CAD build for the part. Positions are in the model's coordinates, mm. Coordinates: 2 decimals unless noted, no trailing zeros. Order: outer loops, then holes, each group sorted by start corner. A loop starts at its lowest first (then second) coordinate and runs counter-clockwise, first axis right, second up. Notation, with made-up numbers: M -28.75,61.25 L -18.75,61.25 A24 cw -18.75,87.25 Z; hole C 86,76 d7. An arc over 180 degrees is marked long. Write item = value, one per line.
from build123d import *

# Parameters (mm, degrees)
CYLINDER115_R          = 1.6
CYLINDER115_DEPTH      = 10
CYLINDER116_R          = 1.6
CYLINDER116_DEPTH      = 10
CYLINDER117_R          = 1.6
CYLINDER117_DEPTH      = 10
CYLINDER114_R          = 1.6
CYLINDER114_DEPTH      = 10
CYLINDER111_R          = 2
CYLINDER111_DEPTH      = 10
CYLINDER110_R          = 2
CYLINDER110_DEPTH      = 10
CYLINDER113_R          = 1.75
CYLINDER113_DEPTH      = 10
CYLINDER112_R          = 1.75
CYLINDER112_DEPTH      = 10
CYLINDER104_R          = 2
CYLINDER104_DEPTH      = 10
CYLINDER105_R          = 2
CYLINDER105_DEPTH      = 10
CYLINDER106_R          = 2
CYLINDER106_DEPTH      = 10
CYLINDER107_R          = 2
CYLINDER107_DEPTH      = 10
CYLINDER109_R          = 24
CYLINDER109_DEPTH      = 7
CYLINDER108_R          = 40
CYLINDER108_DEPTH      = 5
CUT014_PLACEMENT_ANGLE = 1


with BuildPart() as obj1:
    # Cylinder115 → Cylinder115 (new body)
    with BuildSketch(Plane(origin=(40, 0, 65), x_dir=(1, 0, 0), z_dir=(0, 0, 1))):
        Circle(CYLINDER115_R)
    extrude(amount=CYLINDER115_DEPTH)


with BuildPart() as obj2:
    # Cylinder116 → Cylinder116 (new body)
    with BuildSketch(Plane(origin=(5, 35, 65), x_dir=(1, 0, 0), z_dir=(0, 0, 1))):
        Circle(CYLINDER116_R)
    extrude(amount=CYLINDER116_DEPTH)


with BuildPart() as obj3:
    # Cylinder117 → Cylinder117 (new body)
    with BuildSketch(Plane(origin=(5, -35, 65), x_dir=(1, 0, 0), z_dir=(0, 0, 1))):
        Circle(CYLINDER117_R)
    extrude(amount=CYLINDER117_DEPTH)


with BuildPart() as fusion037:
    # Cylinder114 → Cylinder114 (new body)
    with BuildSketch(Plane(origin=(-30, 0, 65), x_dir=(1, 0, 0), z_dir=(0, 0, 1))):
        Circle(CYLINDER114_R)
    extrude(amount=CYLINDER114_DEPTH)

    # Fusion037: union obj1, obj2, obj3
    add(obj1.part)
    add(obj2.part)
    add(obj3.part)


with BuildPart() as wirecut007:
    # Cylinder111 → Cylinder111 (new body)
    with BuildSketch(Plane(origin=(15, 0, 70), x_dir=(1, 0, 0), z_dir=(0, 0, 1))):
        Circle(CYLINDER111_R)
    extrude(amount=CYLINDER111_DEPTH)


with BuildPart() as wirecuts003:
    # Cylinder110 → Cylinder110 (new body)
    with BuildSketch(Plane(origin=(-5, 0, 70), x_dir=(1, 0, 0), z_dir=(0, 0, 1))):
        Circle(CYLINDER110_R)
    extrude(amount=CYLINDER110_DEPTH)

    # Fusion033: union wireCUt007
    add(wirecut007.part)


with BuildPart() as m3cuts007:
    # Cylinder113 → Cylinder113 (new body)
    with BuildSketch(Plane(origin=(5, 9, 70), x_dir=(1, 0, 0), z_dir=(0, 0, 1))):
        Circle(CYLINDER113_R)
    extrude(amount=CYLINDER113_DEPTH)


with BuildPart() as m3cute003:
    # Cylinder112 → Cylinder112 (new body)
    with BuildSketch(Plane(origin=(5, -9, 70), x_dir=(1, 0, 0), z_dir=(0, 0, 1))):
        Circle(CYLINDER112_R)
    extrude(amount=CYLINDER112_DEPTH)

    # Fusion034: union m3Cuts007
    add(m3cuts007.part)


with BuildPart() as cylinder104:
    # Cylinder104 → Cylinder104 (new body)
    with BuildSketch(Plane(origin=(0, -21, 0), x_dir=(1, 0, 0), z_dir=(0, 0, 1))):
        Circle(CYLINDER104_R)
    extrude(amount=CYLINDER104_DEPTH)


with BuildPart() as m3heatsetcuts009:
    # Cylinder105 → Cylinder105 (new body)
    with BuildSketch(Plane(origin=(20, -21, 0), x_dir=(1, 0, 0), z_dir=(0, 0, 1))):
        Circle(CYLINDER105_R)
    extrude(amount=CYLINDER105_DEPTH)

    # Fusion030: union Cylinder104
    add(cylinder104.part)


with BuildPart() as m3heatsetcuts009_1:
    # Fusion030 placement: moved
    add(m3heatsetcuts009.part.moved(Location((-5, 38.5, 70))))


with BuildPart() as cylinder106:
    # Cylinder106 → Cylinder106 (new body)
    with BuildSketch(Plane(origin=(0, -21, 0), x_dir=(1, 0, 0), z_dir=(0, 0, 1))):
        Circle(CYLINDER106_R)
    extrude(amount=CYLINDER106_DEPTH)


with BuildPart() as basecuts003:
    # Cylinder107 → Cylinder107 (new body)
    with BuildSketch(Plane(origin=(20, -21, 0), x_dir=(1, 0, 0), z_dir=(0, 0, 1))):
        Circle(CYLINDER107_R)
    extrude(amount=CYLINDER107_DEPTH)

    # Fusion031: union Cylinder106
    add(cylinder106.part)


with BuildPart() as basecuts003_1:
    # Fusion031 placement: moved
    add(basecuts003.part.moved(Location((-5, 3.5, 70))))

    # Fusion032: union m3HeatSetCuts009
    add(m3heatsetcuts009_1.part)

    # Fusion035: union wireCuts003, m3Cute003
    add(wirecuts003.part)
    add(m3cute003.part)


with BuildPart() as basecut003:
    # Cylinder109 → Cylinder109 (new body)
    with BuildSketch(Plane(origin=(5, 0, 74), x_dir=(1, 0, 0), z_dir=(0, 0, 1))):
        Circle(CYLINDER109_R)
    extrude(amount=CYLINDER109_DEPTH)


with BuildPart() as cut012:
    # Sphere004 → Sphere004 (revolve)
    with BuildSketch(Plane(origin=(5, 0, 74), x_dir=(1, 0, 0), z_dir=(0, -1, 0))):
        with BuildLine():
            ThreePointArc((29, 0), (28.841135, 3.031325), (28.36628, 6.029439))
            Line((28.36628, 6.029439), (0, 6.029439))
            Line((0, 6.029439), (0, 0))
            Line((0, 0), (29, 0))
        make_face()
    revolve(axis=Axis((5, 0, 74), (0, 0, 1)))

    # Cut012: cut baseCut003
    add(basecut003.part, mode=Mode.SUBTRACT)


with BuildPart() as lightmodule003:
    # Cylinder108 → Cylinder108 (new body)
    with BuildSketch(Plane(origin=(5, 0, 70), x_dir=(1, 0, 0), z_dir=(0, 0, 1))):
        Circle(CYLINDER108_R)
    extrude(amount=CYLINDER108_DEPTH)

    # Fusion036: union Cut012
    add(cut012.part)

    # Cut013: cut baseCUts003
    add(basecuts003_1.part, mode=Mode.SUBTRACT)

    # Cut014: cut Fusion037
    add(fusion037.part, mode=Mode.SUBTRACT)


with BuildPart() as lightmodule003_1:
    # Cut014 placement: moved
    add(lightmodule003.part.moved(Location((-46.5, -276, 0))).rotate(Axis((-46.5, -276, 0), (0, 1, 0)), CUT014_PLACEMENT_ANGLE))


solid = lightmodule003_1.part
(1) Slice it at B-B, the plane y = -245. Write the cut outline in (x, z).
Evaluation:
outline = M -65.55,70.34 L -15,69.46 L -14.92,74.46 L -65.47,75.34 Z
(2) Pin check, flat tips, straight feed: pin 1 Ø4 at (y, z) = (-283.5, 79) entering from +X; pin 2 Ø2 at (y, z) = (-305, 72.5) entering from -X; pin 3 Ø1.5 at (y, z) = (-256, 77.5) entering from +X. Stop position of each tip, or through.
Evaluation:
pin_1 = -12.08
pin_2 = -68.8
pin_3 = -18.81
(3) Wall check: line 1 (Y direction, x = -51.5, z = 70.25); line 2 (X direction, y = -257.5, z = 73); line 3 (X direction, y = -270, z = 77.5). Give the ranges that are in metal, low to high. Write a range as from..to.
Evaluation:
line_1 = -314.39..-295.08, -291.92..-277.58, -274.42..-260.08, -256.92..-237.61
line_2 = -75.7..-51.96, -48.49..-31.96, -28.49..-4.75
line_3 = -68.35..-63.39, -16.91..-12.07
(4) Slice it at A-A, the plane z = 72.75. State how many separate pieces and enclosed holes the cut face has, then the cut area to 3 significant figures.
Evaluation:
separate_pieces = 1
enclosed_holes = 12
area = 4,900 mm²
(5) Pull direction X, two halves, no side cores. Call faces 1 (the face through (-48.906, -315.049, 72.518)), 2 (the face through (-51.82, -294.72, 72.57)): +X half, -X half, draft (parallel to the pull), parting line (faces both ways), or undercut.
Evaluation:
face_1 = parting line
face_2 = undercut
